Print and shaded views of the part. All mm, measured from the part's lowest x, y and z. A direction names the side the tool comes from. Round coordinates to 2 decimals unless told otherwise and drop trailing zeros. Loops run counter-clockwise (first coordinate to the right, second up) from the corner with the lowest first, then second, coordinate; pieces in that order, holes last. Notation, with made-up numbers: (-14, 62.25) -> (30, 62.25) arc R21 ccw to (30, 95.25) -> close; hole circle Ø6 at (27.5, 77). An arc over 180 degrees is marked (long way). Use a Markdown table: item, result.
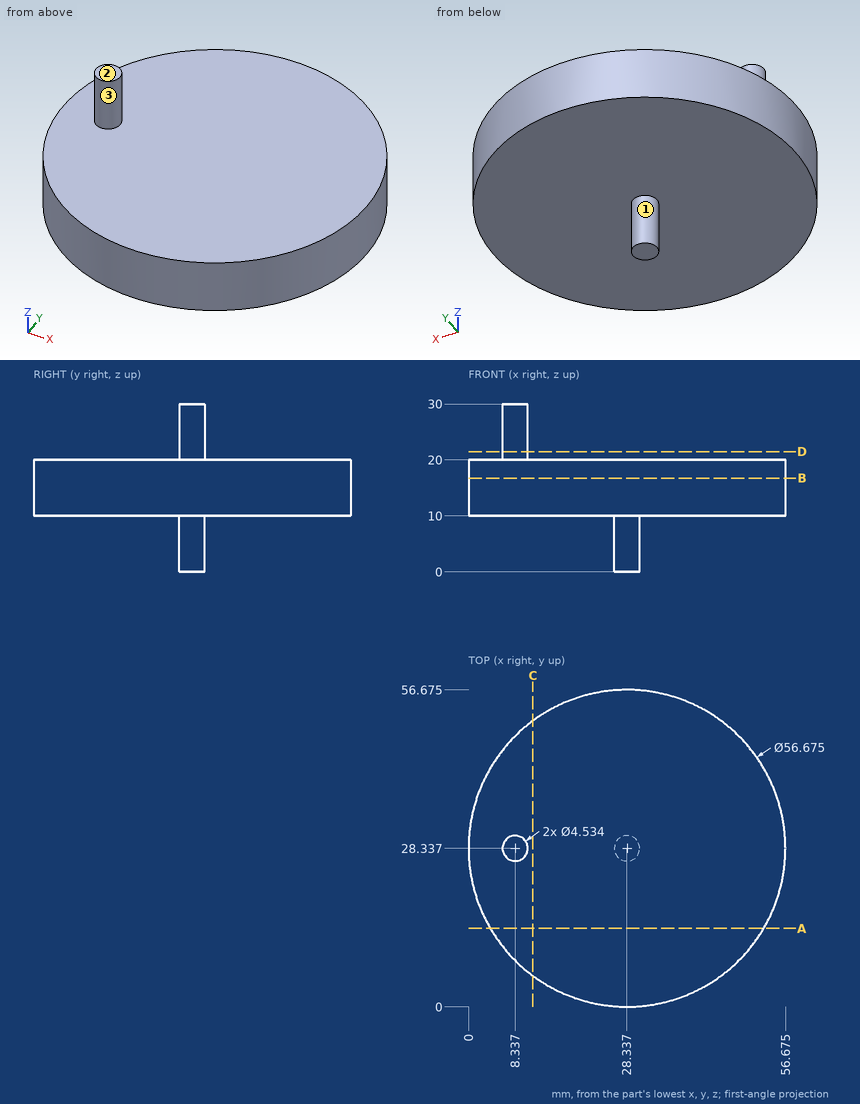
Q1. Flat gauge pins, fed straight in: pin 1 (8 mm diameter, centred on y = 21.5, z = 8, fed in from +X); pin 2 (1.5 mm diameter, centred on y = 29, z = 25.5, fed in from +X); pin 3 (6 mm diameter, centred on x = 43.5, z = 20.5, fed in from +Y). Where does each tip first touch, or does it go through?
Results list:
| item | result |
|---|---|
| pin 1 | stops at x = 56.47 |
| pin 2 | stops at x = 10.6 |
| pin 3 | stops at y = 53.91 |
Q2. Band-saw the part on C-C, the plane x = 11.5. Give the cut face in (y, z) (1 decimal).
Results list:
| item | result |
|---|---|
| outline | (5.5, 10) -> (51.1, 10) -> (51.1, 20) -> (5.5, 20) -> close |
Q3. Band-saw the part on A-A, the plane y = 14. Give the cut face in (x, z) (1 decimal).
Results list:
| item | result |
|---|---|
| outline | (3.9, 10) -> (52.8, 10) -> (52.8, 20) -> (3.9, 20) -> close |
Q4. Band-saw the part on B-B, the plane z = 16.75. Give the cut face in (x, y) (1 decimal).
Results list:
| item | result |
|---|---|
| outline | circle Ø56.7 at (28.3, 28.3) |
Q5. Tool access for the marked faces 1, 2 and 3: list every direction of +Z, -Z, +X, -X, +Y, -Y with a clear straight run to the whole face (end or side of a thin tool).
Results list:
| item | result |
|---|---|
| face 1 | -Z |
| face 2 | +Z, +X, -X, +Y, -Y |
| face 3 | +Z |
Q6. Band-saw the part on D-D, the plane z = 21.5. Give the cut face in (x, y) (1 decimal).
Results list:
| item | result |
|---|---|
| outline | circle Ø4.5 at (8.3, 28.3) |
Q7. Drill centre lines: L1, parallel to Z at x = 46.5, y = 42; L2, parallel to Z at x = 10.5, y = 28.5; L3, parallel to Y at x = 41, z = 16 (1 decimal). Where is each one in solid material? Low to high. Write a range as from..to.
Results list:
| item | result |
|---|---|
| L1 | z = 10..20 |
| L2 | z = 10..30 |
| L3 | y = 3..53.7 |
